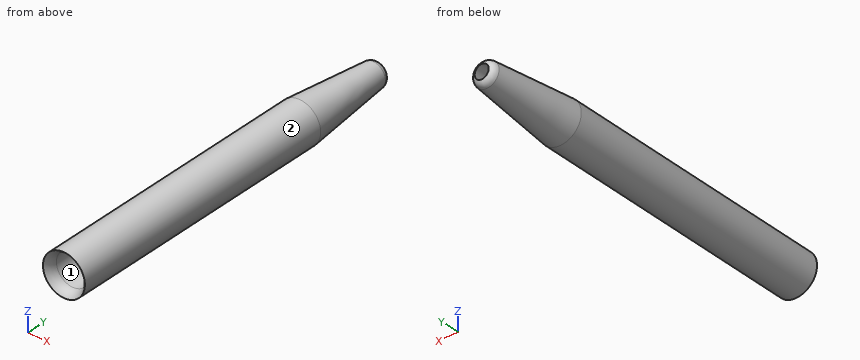
from build123d import *

# Parameters (mm, degrees)
SKETCH1_R           = 9
BOSS_EXTRUDE1_DEPTH = 120
SKETCH2_R           = 7
CUT_EXTRUDE1_DEPTH  = 120
FILLET5_R           = 3
FILLET6_R           = 6


with BuildPart() as part:
    # Sketch1 → Boss-Extrude1 (new body)
    with BuildSketch(Plane(origin=(0, 0, 0), x_dir=(1, 0, 0), z_dir=(0, 1, 0))):
        with Locations(Location((0, 0, 0), (0, 0, 270))):
            Circle(SKETCH1_R)
    extrude(amount=BOSS_EXTRUDE1_DEPTH)

    # Sketch2 → Cut-Extrude1 (cut)
    with BuildSketch(Plane.XZ):
        with Locations(Location((0, 0, 0), (0, 0, 270))):
            Circle(SKETCH2_R)
    extrude(amount=-CUT_EXTRUDE1_DEPTH, mode=Mode.SUBTRACT)

    # Sketch3 → Revolve1 (revolve)
    with BuildSketch(Plane.XY, mode=Mode.PRIVATE) as revolve1_sk:
        Polygon((9, 120), (4.9999999999999964, 160), (2.999999999999999, 160), (6.999999999999999, 120), align=None)
    revolve(revolve1_sk.sketch.rotate(Axis((0, 0, 0), (0, 1, 0)), 90), axis=Axis((0, 0, 0), (0, 1, 0)))

    # Fillet5
    # the kernel refuses this fillet: 3 mm, written as the material it takes off along each edge
    with BuildSketch(Plane(origin=(0, 160, 0), x_dir=(1.1e-16, 0, -1), z_dir=(1, 0, 1.1e-16))) as fillet5_piece_1:
        with BuildLine():
            CenterArc((2.276174333017459, -2.9113701935372944), FILLET5_R, 5.710593137499507, 70.32758962785506)
            Line((2.9999999999999947, -2.842e-14), (3.014476513339645, 0.0582274038707169))
            ThreePointArc((3.014476513339645, 0.0582274038707169), (3.9999999999999956, 0.06000000000000227), (4.9999999999999964, 0.06000000000000227))
            Line((4.9999999999999964, 0.06000000000000227), (5.0597022314125955, 0.00597022314124729))
            Line((5.0597022314125955, 0.00597022314124729), (5.320988135060026, -2.6068888133330574))
            Line((5.320988135060026, -2.6068888133330574), (5.261285903647427, -2.6128590364743047))
        make_face()
    revolve(axis=Axis((0, 160, 0), (0, 1, 0)), mode=Mode.SUBTRACT)

    # Fillet6
    # the kernel refuses this fillet: 6 mm, written as the material it takes off along each edge
    with BuildSketch(Plane(origin=(0, 0, 0), x_dir=(-1.8e-16, 0, -1), z_dir=(-1, 0, 1.8e-16))) as fillet6_piece_1:
        with BuildLine():
            CenterArc((13, -4.47213595499958), FILLET6_R, 131.81031489577862, 48.18968510422138)
            Line((7, -4.47213595499958), (6.88, -4.47213595499958))
            Line((6.88, -4.47213595499958), (6.88, 0))
            Line((6.88, 0), (7, 0.12))
            ThreePointArc((7, 0.12), (8, 0.12), (8.92, 0.08944271909999159))
            Line((8.92, 0.08944271909999159), (9, 0))
        make_face()
    revolve(axis=Axis((0, 0, 0), (0, -1, 0)), mode=Mode.SUBTRACT)


solid = part.part
Work out the finished part from the listing and answer in its coordinate system (mm). Face numbers are marked on the shaded views. Give positions to 0.01 mm unless a question says otherwise; leave off trailing zeros. Order: outer loops, then holes, each group sorted by start corner. A loop starts at its lowest first (then second) coordinate and runs counter-clockwise, first axis right, second up. Notation, with made-up numbers: (-2, 72) -> (22, 72) arc R16 ccw to (22, 89) -> close; hole circle Ø2 at (21.5, 43.5). An arc over 180 degrees is marked (long way). One line per item, written item: value.
Item 1: Determine the mould class of the marked faces 1 and 2 for opening direction Z: released by +Z, released by -Z, zero draft, split by the parting line, or undercut.
Answer sheet:
face 1: undercut
face 2: split by the parting line
Item 2: Find section B-B, the plane y = 123. Give the vertices of the cut face in (x, z), plus the area to 3 significant figures.
Answer sheet:
outline: circle Ø17.4 at (0, 0); hole circle Ø13.4 at (0, 0)
area: 96.8 mm²
Item 3: Flat-ended cylindrical pins translate along their axes: P1, Ø8, axis at x = -4, z = 6, coming from the +Y side; P2, Ø1, axis at y = 99, z = 4.5, coming from the +X side; P3, Ø2, axis at y = 66, z = 5, coming from the -X side. Find the tip coordinate at first contact, or state that the pin passes through.
Answer sheet:
P1: y = 159.94
P2: x = 8.06
P3: x = -8.06
Item 4: Find section A-A, the plane y = 147.5. Give the vertices of the cut face in (x, z).
Answer sheet:
outline: circle Ø12.5 at (0, 0); hole circle Ø8.5 at (0, 0)
Item 5: Straight lines are drawn through the part: probe 1 along X at (y, z) = (31.5, 0); probe 2 along X at (y, z) = (79.5, 3); probe 3 along Z at (x, y) = (1.25, 24). For each, find the intervals that lie inside material, in ascending order.
Answer sheet:
probe 1: -9 to -7, 7 to 9
probe 2: -8.49 to -6.32, 6.32 to 8.49
probe 3: -8.91 to -6.89, 6.89 to 8.91
